The model under review builds one solid part; all positions refer to its coordinate system, in mm. Face numbers are marked on the shaded views. A direction names the side the tool comes from. Coordinates: 2 decimals unless noted, no trailing zeros. Order: outer loops, then holes, each group sorted by start corner. A loop starts at its lowest first (then second) coordinate and runs counter-clockwise, first axis right, second up. Notation, with made-up numbers: (-24, -29.5) - (35, -29.5) arc R29 ccw to (35, -9.5) - close; hole circle Ø9 at (-29.5, 72). An arc over 180 degrees is marked (long way). Answer in a Markdown table with one row per item.
```python
from build123d import *

# Parameters (mm, degrees)
F1_DEPTH  = 16
F2_W      = 70
F2_H      = 3
F3_DEPTH  = 2
F4_W      = 50
F4_H      = 14
F5_DEPTH  = 2
F6_R      = 1
F9_DEPTH  = 4
F11_DEPTH = 38.001
F13_D     = 4
F14_R     = 3
F14_R_2   = 2
F15_DEPTH = 5
F16_R     = 3


# Not quite as in the source:
# - a pattern or mirror of a feature is missing from the dataset's text; its kind, count and spacing are read off the source's solid


with BuildPart() as f1:
    # F0 (on Front) → F1 (new body)
    with BuildSketch(Plane.XZ):
        with BuildLine():
            Line((94, 11), (0, 11))
            ThreePointArc((0, 11), (-11, 0), (0, -11))
            Line((0, -11), (19, -11))
            ThreePointArc((19, -11), (21.7681124643, -11.8361612201), (23.6103896104, -14.064978646))
            ThreePointArc((23.6103896104, -14.064978646), (52.4378053116, -47.6260855158), (95.4479042723, -57.9942665386))
            ThreePointArc((95.4479042723, -57.9942665386), (101.6870615127, -58.9476250352), (106.8734428361, -62.5444881493))
            Line((106.8734428361, -62.5444881493), (108.1694222725, -61))
            ThreePointArc((108.1694222725, -61), (102.3002117906, -57.039668375), (95.2965735981, -56))
            ThreePointArc((95.2965735981, -56), (53.4811996085, -45.9198240056), (25.4545454545, -13.2909701044))
            ThreePointArc((25.4545454545, -13.2909701044), (22.87535745, -10.1706257081), (19, -9))
            Line((19, -9), (0, -9))
            ThreePointArc((0, -9), (-9, 0), (0, 9))
            Line((0, 9), (94, 9))
            Line((94, 9), (94, 11))
        make_face()
    extrude(amount=F1_DEPTH)

    # F2 (on face) → F3 (join)
    with BuildSketch(Plane.XY.offset(11)):
        with Locations((59, -17.5)):
            Rectangle(F2_W, F2_H)
    extrude(amount=-F3_DEPTH)

    # F4 (on face) → F5 (join)
    with BuildSketch(Plane.XZ.offset(19)):
        with Locations((69, 2)):
            Rectangle(F4_W, F4_H)
    extrude(amount=-F5_DEPTH)

    # F6
    f6_edges = [f1.edges().sort_by_distance(p)[0] for p in [
        (59, -19, 11),
        (69, -17, 9),
    ]]
    fillet(f6_edges, radius=F6_R)

    # F7: F1 across plane


with BuildPart() as f1_1:
    add(f1.part)
    add(f1.part.mirror(Plane.XZ))

    # F8 (on face) → F9 (cut)
    with BuildSketch(Plane.XY.offset(11)):
        with BuildLine():
            Line((94, 12), (34, 12))
            ThreePointArc((34, 12), (22, 0), (34, -12))
            Line((34, -12), (94, -12))
            Line((94, -12), (94, 12))
        make_face()
    extrude(amount=-F9_DEPTH, mode=Mode.SUBTRACT)

    # F10 (on face) → F11 (cut, through all)
    with BuildSketch(Plane.XZ.offset(19)):
        with BuildLine():
            ThreePointArc((70, -0.5), (73, 2.5), (70, 5.5))
            Line((70, 5.5), (50, 5.5))
            ThreePointArc((50, 5.5), (47, 2.5), (50, -0.5))
            Line((50, -0.5), (70, -0.5))
        make_face()
    extrude(amount=-F11_DEPTH, mode=Mode.SUBTRACT)

    # F13 (through all)
    with Locations(Plane.XZ.offset(19)):
        with Locations((80, 1)):
            Hole(F13_D / 2)

    # F14 (on face) → F15 (join)
    with BuildSketch(Plane(origin=(0, -17, 0), x_dir=(-1, 0, 0), z_dir=(0, 1, 0))):
        with Locations((-80, 1)):
            Circle(F14_R)
        with Locations((-80, 1)):
            Circle(F14_R_2, mode=Mode.SUBTRACT)
    f15 = extrude(amount=F15_DEPTH)

    # F15_copies: F15 across plane
    add(f15.mirror(Plane.ZX))

    # F16
    f16_edges = [f1_1.edges().sort_by_distance(p)[0] for p in [
        (94, 18, -5),
        (44, 18, -5),
        (94, -18, -5),
        (44, -18, -5),
    ]]
    fillet(f16_edges, radius=F16_R)


solid = f1_1.part
```
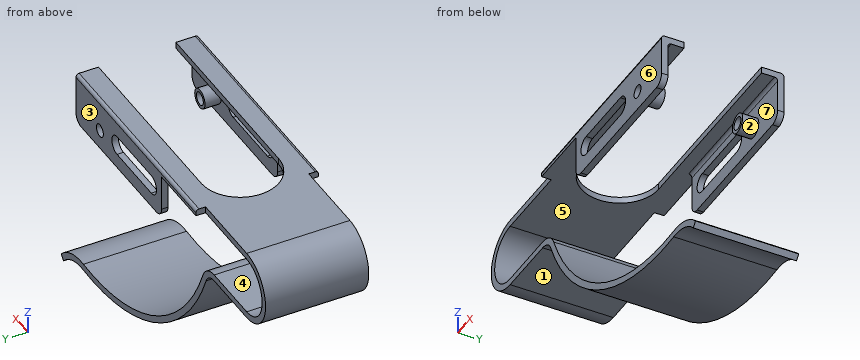
Item 1: We need section D-D, the plane y = -8. Write out the cut boundary in (x, z), then the cut area to 3 significant figures.
Check values:
| item | result |
|---|---|
| outline | (0, -11) - (19, -11) arc R5 cw to (23.61, -14.06) arc R72 ccw to (95.45, -57.99) arc R14 cw to (106.87, -62.54) - (108.17, -61) arc R16 ccw to (95.3, -56) arc R70 cw to (25.45, -13.29) arc R7 ccw to (19, -9) - (0, -9) arc R9 cw to (0, 9) - (25.06, 9) - (25.06, 11) - (0, 11) arc R11 ccw to start |
| area | 369 mm^2 |
Item 2: Mouldability with a two-part tool opening along Y and no side actions: class the marked faces 4, 5, 6 and 7 as +Y half, -Y half, draft (parallel to the pull), parting line (faces both ways), or undercut.
Check values:
| item | result |
|---|---|
| face 4 | draft |
| face 5 | undercut |
| face 6 | -Y half |
| face 7 | undercut |
Item 3: We need section B-B, the plane x = 2. Write out the cut boundary in (y, z).
Check values:
| item | result |
|---|---|
| outline | (-16, -11) - (16, -11) - (16, -9) - (-16, -9) - close; (-16, 9) - (16, 9) - (16, 11) - (-16, 11) - close |
Item 4: Tool access review of the marked faces 1, 2 and 3: name each direction out of +Z, -Z, +X, -X, +Y, -Y from which nothing blocks a thin tool from reaching the whole face with its end or side.
Check values:
| item | result |
|---|---|
| face 1 | -Z, -X, +Y, -Y |
| face 2 | none |
| face 3 | +Z, -Z, +X, -X, +Y |
Item 5: We need section C-C, the plane x = 71.5. Write out the cut boundary in (y, z), then the cut area to 3 significant figures.
Check values:
| item | result |
|---|---|
| outline | (-19, -5) - (-17, -5) - (-17, -0.1) - (-19, -0.1) - close; (-19, 5.1) - (-17, 5.1) - (-17, 8) arc R1 cw to (-16, 9) - (-12, 9) - (-12, 11) - (-18, 11) arc R1 ccw to (-19, 10) - close; (-16, -55.78) - (16, -55.78) - (16, -53.71) - (-16, -53.71) - close; (12, 9) - (16, 9) arc R1 cw to (17, 8) - (17, 5.1) - (19, 5.1) - (19, 10) arc R1 ccw to (18, 11) - (12, 11) - close; (17, -5) - (19, -5) - (19, -0.1) - (17, -0.1) - close |
| area | 130 mm^2 |
Item 6: Clearance check with flat-ended pins moving along their axes: pin 1 Ø1 at (x, y) = (61.5, 18.5) entering from -Z; pin 2 Ø1.6 at (y, z) = (-18, 10) entering from -X; pin 3 Ø3.5 at (y, z) = (16.5, 3.5) entering from +X; pin 4 Ø3 at (x, z) = (54.5, -44.5) entering from +Y. State where each tip first meets the part, or that it passes through.
Check values:
| item | result |
|---|---|
| pin 1 | z = -5 |
| pin 2 | x = 24 |
| pin 3 | x = 94 |
| pin 4 | through |
Item 7: We need section A-A, the plane y = -13.5. Write out the cut boundary in (x, z), then the cut area to 3 significant figures.
Check values:
| item | result |
|---|---|
| outline | (0, -11) - (19, -11) arc R5 cw to (23.61, -14.06) arc R72 ccw to (95.45, -57.99) arc R14 cw to (106.87, -62.54) - (108.17, -61) arc R16 ccw to (95.3, -56) arc R70 cw to (25.45, -13.29) arc R7 ccw to (19, -9) - (0, -9) arc R9 cw to (0, 9) - (94, 9) - (94, 11) - (0, 11) arc R11 ccw to start; circle Ø6 at (80, 1); hole circle Ø4 at (80, 1) |
| area | 523 mm^2 |
Item 8: To check wall thickness, follow line 1 (Z direction, x = 80, y = -17.8); line 2 (Z direction, x = 80, y = -15); line 3 (Y direction, x = 57.5, z = -4). State the ranges of each line that lie inside material, in increasing order. Write a range as from..to.
Check values:
| item | result |
|---|---|
| line 1 | -5..-1, 3..11 |
| line 2 | -57.5..-55.48, -2..-1, 3..4, 9..11 |
| line 3 | -19..-17, 17..19 |
